Job drawing, mm, ordinate dimensions from the low corner. One solid piece. A direction names the side the tool comes from. Round coordinates to 2 decimals unless told otherwise and drop trailing zeros. Loops run counter-clockwise (first coordinate to the right, second up) from the corner with the lowest first, then second, coordinate; pieces in that order, holes last.
1) Mould opens along X. For the marked faces 1, 2 and 3 say: +X half, -X half, draft (parallel to the pull), parting line (faces both ways), or undercut.
2) Band-saw the part on A-A, the plane x = 48.26. Write the cut outline in (y, z) (3 decimals).
3) Probe line 1 (X direction, y = 47.6, z = 48.26); line 2 (X direction, y = 5, z = 71) (3 decimals); line 3 (Z direction, x = 48, y = 47). List the from-to ranges inside material, lowest first.
4) Band-saw the part on C-C, the plane y = 9. Write the cut outline in (x, z) (3 decimals), then the cut area to 3 significant figures.
5) Band-saw the part on B-B, the plane z = 48.26. Write the cut outline in (x, y) (3 decimals).
6) 3-axis set-ups, long thin cutter, end or side, ignore diameter. For the marked faces 4, 5, 6, 7 and 8: which of +Z, -Z, +X, -X, +Y, -Y reach the whole face in a straight line?
7) Drop flat-ended pins along their axis: P1, Ø6, axis at x = 44.5, z = 59, coming from the -Y side; P2, Ø4, axis at x = 30, y = 37.5, coming from the -Z side; P3, Ø13.5, axis at x = 46, y = 12, coming from the +Z side. Give the stop position or say it passes through.
8) Band-saw the part on D-D, the plane z = 78. Write the cut outline in (x, y) (3 decimals).
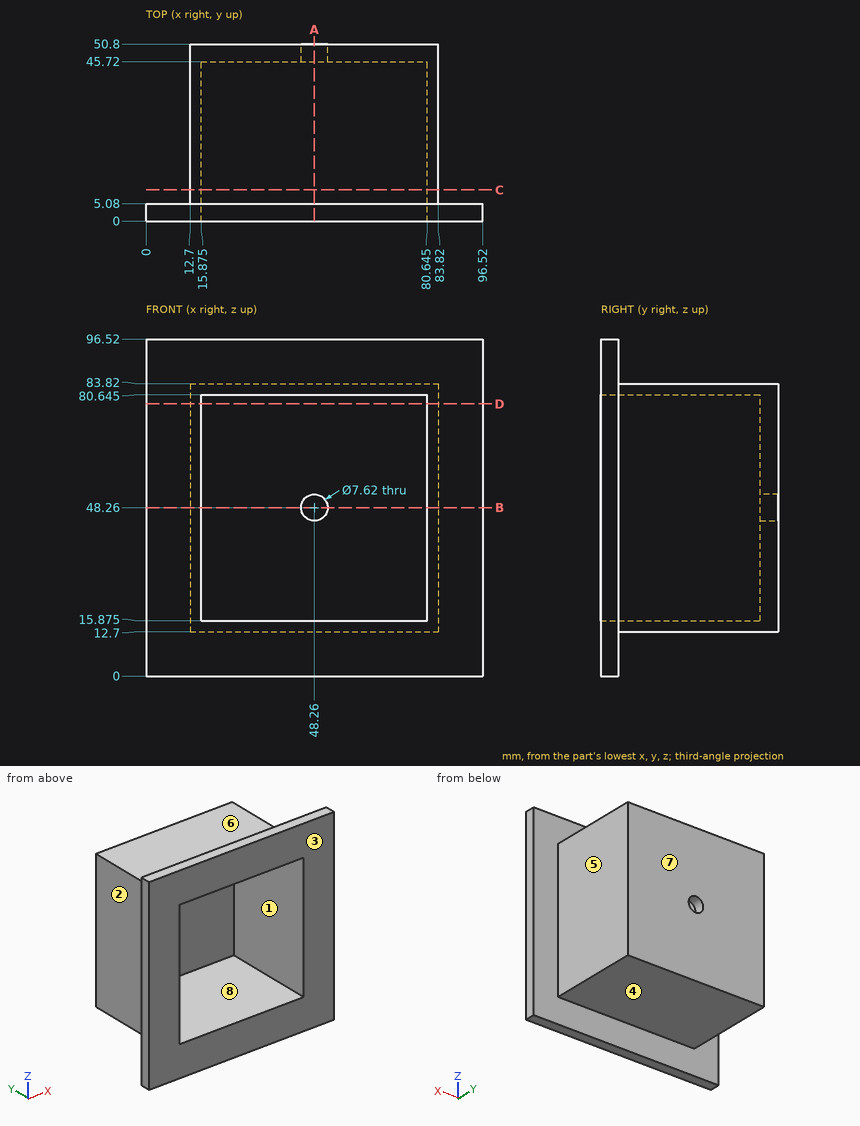
Reported:
1. face 1: undercut
1. face 2: -X half
1. face 3: draft
2. outline: (0, 0) - (5.08, 0) - (5.08, 12.7) - (50.8, 12.7) - (50.8, 44.45) - (45.72, 44.45) - (45.72, 15.875) - (0, 15.875) - close; (0, 80.645) - (45.72, 80.645) - (45.72, 52.07) - (50.8, 52.07) - (50.8, 83.82) - (5.08, 83.82) - (5.08, 96.52) - (0, 96.52) - close
3. line 1: x = 12.7 to 44.45, 52.07 to 83.82
3. line 2: x = 0 to 15.875, 80.645 to 96.52
3. line 3: z = 12.7 to 44.46, 52.06 to 83.82
4. outline: (12.7, 12.7) - (83.82, 12.7) - (83.82, 83.82) - (12.7, 83.82) - close; hole (15.875, 15.875) - (80.645, 15.875) - (80.645, 80.645) - (15.875, 80.645) - close
4. area: 863 mm2
5. outline: (0, 0) - (15.875, 0) - (15.875, 45.72) - (44.45, 45.72) - (44.45, 50.8) - (12.7, 50.8) - (12.7, 5.08) - (0, 5.08) - close; (52.07, 45.72) - (80.645, 45.72) - (80.645, 0) - (96.52, 0) - (96.52, 5.08) - (83.82, 5.08) - (83.82, 50.8) - (52.07, 50.8) - close
6. face 4: -Z, +X, -X, +Y
6. face 5: +Z, -Z, +X, +Y
6. face 6: +Z, +X, -X, +Y
6. face 7: +Z, -Z, +X, -X, +Y
6. face 8: -Y
7. P1: stops at y = 45.72
7. P2: stops at z = 12.7
7. P3: stops at z = 83.82
8. outline: (0, 0) - (15.875, 0) - (15.875, 45.72) - (80.645, 45.72) - (80.645, 0) - (96.52, 0) - (96.52, 5.08) - (83.82, 5.08) - (83.82, 50.8) - (12.7, 50.8) - (12.7, 5.08) - (0, 5.08) - close
